Part model, mm, in its own coordinate system. Face numbers are marked on the shaded views. A direction names the side the tool comes from. Round coordinates to 2 decimals unless told otherwise and drop trailing zeros. Loops run counter-clockwise (first coordinate to the right, second up) from the corner with the lowest first, then second, coordinate; pieces in that order, holes last. Notation, with made-up numbers: (10, -29) - (34, -29) arc R27 cw to (34, -3) - close; hole circle Ø7 at (17, 3). An arc over 180 degrees is marked (long way). Write each question's results on one line, items separated by ' | '. Start each with the question number.
(1) Tool access for the marked faces 5, 6 and 7: list every direction of +Z, -Z, +X, -X, +Y, -Y with a clear straight run to the whole face (end or side of a thin tool).
(2) Drill centre lines: L1, parallel to Z at x = -32, y = -12; L2, parallel to Y at x = 12, z = -21.5; L3, parallel to Y at x = -16.5, z = -71.5. Where is each one in solid material? Low to high.
(3) Cut at C-C, the plane y = -21. List the corners of the cut face in (x, z), then the cut area to 3 significant figures.
(4) Flat gauge pins, fed straight in: P1, Ø3, axis at x = -35, y = 20, coming from the -Z side; P2, Ø3, axis at x = -46, z = -33, coming from the +Y side; P3, Ø3, axis at y = 22.5, z = -15.5, coming from the -X side. Where does each tip first touch, or does it go through?
(5) Mould opens along Y. For the marked faces 1, 2, 3 and 4 say: released by +Y, released by -Y, zero draft, split by the parting line, or undercut.
(6) Cut at A-A, the plane x = -2. List the corners of the cut face in (y, z).
(7) Cut at B-B, the plane z = -45. List the corners of the cut face in (x, y).
(8) Cut at D-D, the plane z = -16. List the corners of the cut face in (x, y), then the cut area to 3 significant figures.
from build123d import *

# Parameters (mm, degrees)
F0_W     = 76.2
F0_H     = 76.2
F1_DEPTH = 76.2
F2_R     = 5.08
F3_T     = -2.54
F4_W     = 49.854696
F4_H     = 36.147542
F5_DEPTH = 25.4


with BuildPart() as f1:
    # F0 (on Top) → F1 (new body)
    with BuildSketch(Plane.XY):
        Rectangle(F0_W, F0_H)
    extrude(amount=-F1_DEPTH)

    # F2
    f2_edges = [f1.edges().sort_by_distance(p)[0] for p in [
        (0, -38.1, 0),
        (0, 38.1, 0),
        (0, -38.1, -76.2),
        (0, 38.1, -76.2),
        (-38.1, 0, -76.2),
        (-38.1, 38.1, -38.1),
        (-38.1, 0, 0),
        (-38.1, -38.1, -38.1),
    ]]
    fillet(f2_edges, radius=F2_R)

    # F3
    f3_openings = [f1.faces().sort_by_distance(p)[0] for p in [
        (38.1, 0, -38.1),
    ]]
    offset(amount=F3_T, openings=f3_openings)

    # F4 (on face) → F5 (join)
    with BuildSketch(Plane(origin=(-38.1, 0, 0), x_dir=(0, -1, 0), z_dir=(-1, 0, 0))):
        with Locations((0.608757, -36.575835)):
            Rectangle(F4_W, F4_H)
    extrude(amount=F5_DEPTH)


solid = f1.part
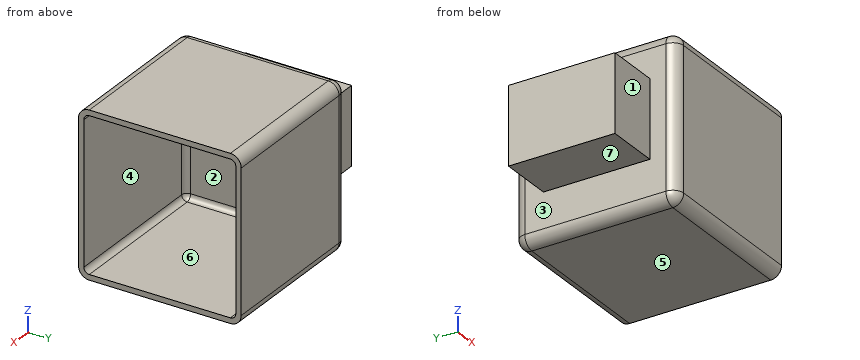
A:
1) face 5: -Z, +X, -X, +Y, -Y | face 6: +X | face 7: -Z, -X, +Y, -Y
2) L1: -76.2 to -73.66, -2.54 to 0 | L2: -38.1 to -35.56, 35.56 to 38.1 | L3: -38.09 to -35.53, 35.53 to 38.09
3) outline: (-63.5, -54.65) - (-38.1, -54.65) - (-38.1, -71.12) arc R5.08 ccw to (-33.02, -76.2) - (38.1, -76.2) - (38.1, -73.66) - (-33.02, -73.66) arc R2.54 cw to (-35.56, -71.12) - (-35.56, -5.08) arc R2.54 cw to (-33.02, -2.54) - (38.1, -2.54) - (38.1, 0) - (-33.02, 0) arc R5.08 ccw to (-38.1, -5.08) - (-38.1, -18.5) - (-63.5, -18.5) - close | area: 1,480 mm2
4) P1: z = -76.18 | P2: y = 24.32 | P3: x = -38.1
5) face 1: released by -Y | face 2: undercut | face 3: zero draft | face 4: undercut
6) outline: (-38.1, -71.12) arc R5.08 ccw to (-33.02, -76.2) - (33.02, -76.2) arc R5.08 ccw to (38.1, -71.12) - (38.1, -5.08) arc R5.08 ccw to (33.02, 0) - (-33.02, 0) arc R5.08 ccw to (-38.1, -5.08) - close; hole (-35.56, -71.12) arc R2.54 ccw to (-33.02, -73.66) - (33.02, -73.66) arc R2.54 ccw to (35.56, -71.12) - (35.56, -5.08) arc R2.54 ccw to (33.02, -2.54) - (-33.02, -2.54) arc R2.54 ccw to (-35.56, -5.08) - close
7) outline: (-63.5, -25.54) - (-38.1, -25.54) - (-38.1, -33.02) arc R5.08 ccw to (-33.02, -38.1) - (38.1, -38.1) - (38.1, -35.56) - (-33.02, -35.56) arc R2.54 cw to (-35.56, -33.02) - (-35.56, 33.02) arc R2.54 cw to (-33.02, 35.56) - (38.1, 35.56) - (38.1, 38.1) - (-33.02, 38.1) arc R5.08 ccw to (-38.1, 33.02) - (-38.1, 24.32) - (-63.5, 24.32) - close
8) outline: (-38.1, -33.02) arc R5.08 ccw to (-33.02, -38.1) - (38.1, -38.1) - (38.1, -35.56) - (-33.02, -35.56) arc R2.54 cw to (-35.56, -33.02) - (-35.56, 33.02) arc R2.54 cw to (-33.02, 35.56) - (38.1, 35.56) - (38.1, 38.1) - (-33.02, 38.1) arc R5.08 ccw to (-38.1, 33.02) - close | area: 559 mm2
